Autodesk Inventor part; units mm, degrees
ref_plane "YZ Plane" through (0, 0, 0) normal (1, 0, 0) x (0, 1, 0)
ref_plane "XZ Plane" through (0, 0, 0) normal (0, 1, 0) x (-1, 0, 0)
ref_plane "XY Plane" through (0, 0, 0) normal (0, 0, 1) x (1, 0, 0)
sketch "Sketch1" plane through (0, 0, 0) normal (0, 1, 0) x (-1, 0, 0)
  line L0 (0, 0) -> (0, -288.984) construction
  line L1 (5, 0) -> (5, -288.984)
  line L2 (-5, -288.984) -> (-5, 0)
  arc A0 (5, 0) -> (-5, 0) centre (0, 0) ccw
  arc A1 (-5, -288.984) -> (5, -288.984) centre (0, -288.984) ccw
  circle A2 centre (0, 0) radius 1.65
  circle A3 centre (0, -288.984) radius 1.65
  circle A4 centre (0, -231.585) radius 1.65
  arc A5 (-5, -231.585) -> (-5, 0) centre (-593.7207, -115.7925) ccw
  arc A6 (5, -231.585) -> (5, 0) centre (-583.7207, -115.7925) ccw
  point P0 (0, -144.492)
  dimension "d0" = 3.3
  dimension "d1" = 3.3
  dimension "d2" = 10
  dimension "d3" = 288.984
  dimension "d14" = 3.3
  dimension "d15" = 231.585
  dimension "d18" = 600
  dimension "d19" = 600
extrude "Extrusion1" add sketch "Sketch1" along normal blind 6 contours L1 A1 L2 A5 | L1 A5 A6 | L1 A5 A0
sketch "Sketch2" plane through (0, 6, 0) normal (0, 1, 0) x (1, 0, 0)
  line L0 (-27.7109, 299.4385) -> (14.5069, 299.4385)
  line L1 (14.5069, 299.4385) -> (14.5069, 139.1377)
  line L2 (14.5069, 139.1377) -> (-27.7109, 139.1377)
  line L3 (-27.7109, 139.1377) -> (-27.7109, 299.4385)
  line L4 (-101.0366, 321.0236) -> (54.5028, 321.0236)
  line L5 (54.5028, 321.0236) -> (54.5028, -14.1796)
  line L6 (54.5028, -14.1796) -> (-101.0366, -14.1796)
  line L7 (-101.0366, -14.1796) -> (-101.0366, 321.0236)
  point P0 (0, 0)
extrude "Extrusion2" cut sketch "Sketch2" against normal blind 10
properties part number "Part_7_p2"
Could you check a few things on this model? Use its own coordinates, in mm. A direction names the side the tool comes from. Give positions to 0.01 mm unless a question says otherwise; leave off trailing zeros. Order: outer loops, then holes, each group sorted by start corner. A loop starts at its lowest first (then second) coordinate and runs counter-clockwise, first axis right, second up.
1. I need wall thicknesses on L1, parallel to X at y = 1.6, z = -266.5; L2, parallel to X at y = 4.7, z = -190. Which ranges of each line are inside material? Lowest first, please.
Answers below:
L1: x = -5 to 5
L2: x = -11.67 to -1.67
2. Thinking about a two-plate mould opening in Z: for faces 1 (the flat face through (-3, 0, -215)), 2 (the cylindrical face through (-12.283, 2.958, -184.924)), 3 (the cylindrical face through (0.21, 2.96, -233.22)), which applies, +Z half, -Z half, draft (parallel to the pull), parting line (faces both ways), or undercut?
Answers below:
face 1: draft
face 2: -Z half
face 3: undercut
3. Suppose I cut it at A-A (y = 2.6). State how many separate pieces and enclosed holes the cut face has, plus the area to 3 significant figures.
Answers below:
separate pieces: 1
enclosed holes: 2
area: 1,520 mm2
4. Which directions (+Z, -Z, +X, -X, +Y, -Y) give clear straight access to the entire face, cutting with the end or side of a thin tool? Please do faces 4 (the cylindrical face through (-2.283, 2.958, -184.924)), 5 (the flat face through (-5, 3, -260)).
Answers below:
face 4: +Z, +X, +Y, -Y
face 5: -Z, -X, +Y, -Y
5. Suppose I cut it at C-C (z = -176). Write out the boundary of the cut face in (x, y), plus the area to 3 significant figures.
Answers below:
outline: (-13.25, 0) - (-3.25, 0) - (-3.25, 6) - (-13.25, 6) - close
area: 60.0 mm2
6. Suppose I cut it at D-D (x = -8). Write out the boundary of the cut face in (y, z).
Answers below:
outline: (0, -215.12) - (6, -215.12) - (6, -139.14) - (0, -139.14) - close
7. Suppose I cut it at B-B (x = 0). Write out the boundary of the cut face in (y, z) (3 decimals).
Answers below:
outline: (0, -293.984) - (6, -293.984) - (6, -290.634) - (0, -290.634) - close; (0, -287.334) - (6, -287.334) - (6, -233.235) - (0, -233.235) - close; (0, -229.935) - (6, -229.935) - (6, -202.37) - (0, -202.37) - close
